```python
from build123d import *

# Parameters (mm, degrees)
SKETCH1_W           = 42
SKETCH1_H           = 42
BOSS_EXTRUDE1_DEPTH = 39
CHAMFER1_SIZE       = 4
SKETCH2_R           = 20.95
BOSS_EXTRUDE2_DEPTH = 41.75
SKETCH3_R           = 4
BOSS_EXTRUDE3_DEPTH = 20
CUT_EXTRUDE1_START  = -15
CUT_EXTRUDE1_DEPTH  = 15
SKETCH5_R           = 2
CUT_EXTRUDE2_DEPTH  = 20


with BuildPart() as part:
    # Sketch1 → Boss-Extrude1 (new body)
    with BuildSketch(Plane.XY):
        Rectangle(SKETCH1_W, SKETCH1_H)
    extrude(amount=BOSS_EXTRUDE1_DEPTH)

    # Chamfer1
    chamfer1_edges = [part.edges().sort_by_distance(p)[0] for p in [
        (21, -21, 19.5),
        (-21, -21, 19.5),
        (-21, 21, 19.5),
        (21, 21, 19.5),
    ]]
    chamfer(chamfer1_edges, length=CHAMFER1_SIZE)

    # Sketch2 → Boss-Extrude2 (add)
    with BuildSketch(Plane(origin=(0, 0, 0), x_dir=(-1, 0, 0), z_dir=(0, 0, -1))):
        with Locations(Location((0, 0, 0), (0, 0, 180))):
            Circle(SKETCH2_R)
    extrude(amount=BOSS_EXTRUDE2_DEPTH)

    # Sketch3 → Boss-Extrude3 (add)
    with BuildSketch(Plane(origin=(0, 0, -41.75), x_dir=(-1, 0, 0), z_dir=(0, 0, -1))):
        Circle(SKETCH3_R)
    extrude(amount=BOSS_EXTRUDE3_DEPTH)

    # Sketch4 → Cut-Extrude1 (cut)
    with BuildSketch(Plane(origin=(0, 0, -61.75), x_dir=(-1, 0, 0), z_dir=(0, 0, -1)).offset(CUT_EXTRUDE1_START)):
        with BuildLine():
            Line((-2.645751311, 3), (2.645751311, 3))
            ThreePointArc((2.645751311, 3), (0, 4), (-2.645751311, 3))
        make_face()
    extrude(amount=CUT_EXTRUDE1_DEPTH, mode=Mode.SUBTRACT)

    # Sketch5 → Cut-Extrude2 (cut)
    with BuildSketch(Plane(origin=(0, 0, -41.75), x_dir=(-1, 0, 0), z_dir=(0, 0, -1))):
        with Locations((12.02081528, 12.02081528)):
            Circle(SKETCH5_R)
        with Locations((12.02081528, -12.02081528)):
            Circle(SKETCH5_R)
        with Locations((-12.02081528, -12.02081528)):
            Circle(SKETCH5_R)
        with Locations((-12.02081528, 12.02081528)):
            Circle(SKETCH5_R)
    extrude(amount=-CUT_EXTRUDE2_DEPTH, mode=Mode.SUBTRACT)


solid = part.part
```
Geometry: final body of the model. Coordinates: model frame, mm. A direction names the side the tool comes from. Coordinates: 2 decimals unless noted, no trailing zeros. Order: outer loops, then holes, each group sorted by start corner. A loop starts at its lowest first (then second) coordinate and runs counter-clockwise, first axis right, second up. Notation, with made-up numbers: (13.5, 87.5) -> (27.5, 87.5) arc R35 cw to (27.5, 125.5) -> close; hole circle Ø9 at (54, 2). An arc over 180 degrees is marked (long way). Write item = value, one per line.
(1) Access query for faces 4 (the cylindrical face through (12.454, 10.068, -31.89)), 5 (the flat face through (0, 21, 19)), 6 (the flat face through (0, 3, -54)). Directions: +Z, -Z, +X, -X, +Y, -Y. A direction counts if a zero-diameter tool reaches every point of the face in a straight line with its end or side. Return the directions, or none.
Solved:
face_4 = -Z
face_5 = +Z, -Z, +X, -X, +Y
face_6 = -Z, +X, -X, +Y
(2) Cut plane C-C on z = -14.5. Return loops of the section in (x, y), plus the area to 3 significant figures.
Solved:
outline = circle Ø41.9 at (0, 0)
area = 1,380 mm²
(3) Cut plane A-A on y = 0. Return loops of the section in (x, z), plus the area to 3 significant figures.
Solved:
outline = (-21, 0) -> (-20.95, 0) -> (-20.95, -41.75) -> (-4, -41.75) -> (-4, -61.75) -> (4, -61.75) -> (4, -41.75) -> (20.95, -41.75) -> (20.95, 0) -> (21, 0) -> (21, 39) -> (-21, 39) -> close
area = 3,550 mm²
(4) Pin query (flat end, axial travel): pin 1 Ø2 at (x, y) = (-12, 11.5) entering from -Z; pin 2 Ø4 at (x, z) = (-0.5, -51) entering from +Y; pin 3 Ø4 at (x, y) = (-9.5, -11.5) entering from -Z. Return the tip coordinate at first contact, or that it passes through.
Solved:
pin_1 = -21.75
pin_2 = 3
pin_3 = -41.75
(5) Pull-direction query (Y, two-part tool) for faces 1 (the flat face through (-21, 0, 19)), 2 (the flat face through (-12, 12, -21.75)), 3 (the flat face through (19, -19, 19)); classes: pulls with the +Y half, pulls with the -Y half, needs draft (parallel to the pull), parting line crosses it, or undercut.
Solved:
face_1 = needs draft
face_2 = undercut
face_3 = pulls with the -Y half
(6) Line query: line 1 (X direction, y = -0.5, z = -5.5); line 2 (Z direction, x = -7.5, y = -16); line 3 (Z direction, x = 11, y = 10.5). Output: solid intervals per line, ascending.
Solved:
line_1 = -20.94 to 20.94
line_2 = -41.75 to 39
line_3 = -21.75 to 39
(7) Cut plane D-D on z = -33.5. Return loops of the section in (x, y), plus the area to 3 significant figures.
Solved:
outline = circle Ø41.9 at (0, 0); hole circle Ø4 at (-12.02, -12.02); hole circle Ø4 at (-12.02, 12.02); hole circle Ø4 at (12.02, -12.02); hole circle Ø4 at (12.02, 12.02)
area = 1,330 mm²
(8) Cut plane B-B on x = 0. Return loops of the section in (y, z), plus the area to 3 significant figures.
Solved:
outline = (-21, 0) -> (-20.95, 0) -> (-20.95, -41.75) -> (-4, -41.75) -> (-4, -61.75) -> (3, -61.75) -> (3, -46.75) -> (4, -46.75) -> (4, -41.75) -> (20.95, -41.75) -> (20.95, 0) -> (21, 0) -> (21, 39) -> (-21, 39) -> close
area = 3,530 mm²
